Source: CAD feature listing. Evaluate the final solid. Frame: model axes, mm. Give positions to 0.01 mm unless a question says otherwise; leave off trailing zeros. Order: outer loops, then holes, each group sorted by start corner. A loop starts at its lowest first (then second) coordinate and runs counter-clockwise, first axis right, second up. Notation, with made-up numbers: M 20.25,52 L 39.25,52 A32 ccw 39.25,91 Z; hole C 42,49.5 d3. An arc over 180 degrees is marked long. Answer as a JSON object with one key per item and string values. Group by question number.
1. Section query D-D (z = 5.25). Output: boundary loops of the cut face in (x, y).
2. Section query B-B (x = 16). Output: boundary loops of the cut face in (y, z).
3. Material intervals for L1, parallel to Y at x = -16, z = 1.3; L2, parallel to X at y = 18, z = 0.65; L3, parallel to Y at x = -15.5, z = 0.75, sorted ascending. Write a range as [from, to].
4. Section query A-A (y = 18). Output: boundary loops of the cut face in (x, z).
5. Section query C-C (y = 12.5). Output: boundary loops of the cut face in (x, z), plus the area to 3 significant figures.
6. Pin query (flat end, axial travel): P1, Ø6.5, axis at x = -16, y = -10, coming from the -Z side; P2, Ø3, axis at x = -16, y = 18, coming from the +Z side; P3, Ø3, axis at x = 10, z = 6, coming from the -Y side; P4, Ø11.5, axis at x = -2.5, y = 0.5, coming from the +Z side. Return the tip coordinate at first contact, or that it passes through.
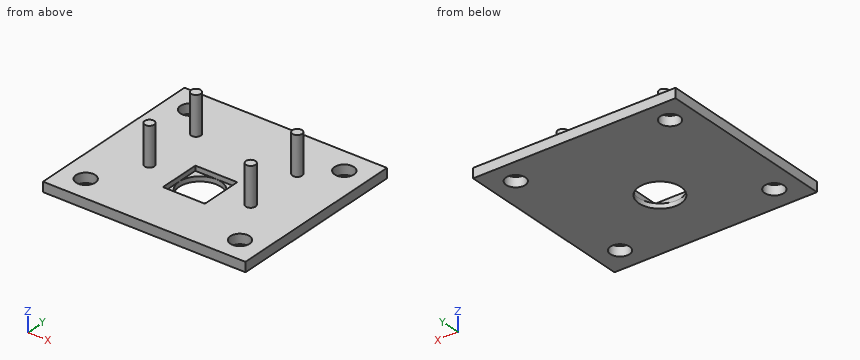
from build123d import *

# Parameters (mm, degrees)
CYLINDER002_R     = 1
CYLINDER002_DEPTH = 10
CYLINDER003_R     = 1
CYLINDER003_DEPTH = 10
CYLINDER004_R     = 1
CYLINDER004_DEPTH = 10
CYLINDER005_R     = 2
CYLINDER005_DEPTH = 10
CYLINDER006_R     = 2
CYLINDER006_DEPTH = 10
CYLINDER007_R     = 2
CYLINDER007_DEPTH = 10
CYLINDER008_R     = 2
CYLINDER008_DEPTH = 10
CYLINDER_R        = 4.35
CYLINDER_DEPTH    = 10
BOX_W             = 8.7
BOX_H             = 8.7
BOX_DEPTH         = 2
BOX001_W          = 42
BOX001_H          = 38
BOX001_DEPTH      = 2
CYLINDER001_R     = 1
CYLINDER001_DEPTH = 10


with BuildPart() as screw_support001:
    # Cylinder002 → Cylinder002 (new body)
    with BuildSketch(Plane(origin=(10.5, 0, 0), x_dir=(1, 0, 0), z_dir=(0, 0, 1))):
        Circle(CYLINDER002_R)
    extrude(amount=CYLINDER002_DEPTH)


with BuildPart() as screw_support002:
    # Cylinder003 → Cylinder003 (new body)
    with BuildSketch(Plane(origin=(-10.5, 12.5, 0), x_dir=(1, 0, 0), z_dir=(0, 0, 1))):
        Circle(CYLINDER003_R)
    extrude(amount=CYLINDER003_DEPTH)


with BuildPart() as screw_support003:
    # Cylinder004 → Cylinder004 (new body)
    with BuildSketch(Plane(origin=(10.5, 12.5, 0), x_dir=(1, 0, 0), z_dir=(0, 0, 1))):
        Circle(CYLINDER004_R)
    extrude(amount=CYLINDER004_DEPTH)


with BuildPart() as bolthole:
    # Cylinder005 → Cylinder005 (new body)
    with BuildSketch(Plane(origin=(-16, -10, 0), x_dir=(1, 0, 0), z_dir=(0, 0, 1))):
        Circle(CYLINDER005_R)
    extrude(amount=CYLINDER005_DEPTH)


with BuildPart() as bolthole001:
    # Cylinder006 → Cylinder006 (new body)
    with BuildSketch(Plane(origin=(16, 18, 0), x_dir=(1, 0, 0), z_dir=(0, 0, 1))):
        Circle(CYLINDER006_R)
    extrude(amount=CYLINDER006_DEPTH)


with BuildPart() as bolthole002:
    # Cylinder007 → Cylinder007 (new body)
    with BuildSketch(Plane(origin=(16, -10, 0), x_dir=(1, 0, 0), z_dir=(0, 0, 1))):
        Circle(CYLINDER007_R)
    extrude(amount=CYLINDER007_DEPTH)


with BuildPart() as bolthole003:
    # Cylinder008 → Cylinder008 (new body)
    with BuildSketch(Plane(origin=(-16, 18, 0), x_dir=(1, 0, 0), z_dir=(0, 0, 1))):
        Circle(CYLINDER008_R)
    extrude(amount=CYLINDER008_DEPTH)


with BuildPart() as cylinder:
    # Cylinder → Cylinder (new body)
    with BuildSketch(Plane.XY.offset(-3)):
        Circle(CYLINDER_R)
    extrude(amount=CYLINDER_DEPTH)


with BuildPart() as cube:
    # Box → Box (new body)
    with BuildSketch(Plane(origin=(-4.35, -4.35, 1), x_dir=(1, 0, 0), z_dir=(0, 0, 1))):
        with Locations((4.35, 4.35)):
            Rectangle(BOX_W, BOX_H)
    extrude(amount=BOX_DEPTH)


with BuildPart() as cut005:
    # Box001 → Box001 (new body)
    with BuildSketch(Plane(origin=(-21, -15, 0), x_dir=(1, 0, 0), z_dir=(0, 0, 1))):
        with Locations((21, 19)):
            Rectangle(BOX001_W, BOX001_H)
    extrude(amount=BOX001_DEPTH)

    # Cut: cut Cube
    add(cube.part, mode=Mode.SUBTRACT)

    # Cut001: cut Cylinder
    add(cylinder.part, mode=Mode.SUBTRACT)

    # Cut002: cut BoltHole003
    add(bolthole003.part, mode=Mode.SUBTRACT)

    # Cut003: cut BoltHole002
    add(bolthole002.part, mode=Mode.SUBTRACT)

    # Cut004: cut BoltHole001
    add(bolthole001.part, mode=Mode.SUBTRACT)

    # Cut005: cut BoltHole
    add(bolthole.part, mode=Mode.SUBTRACT)


with BuildPart() as fusion_camfront:
    # Cylinder001 → Cylinder001 (new body)
    with BuildSketch(Plane(origin=(-10.5, 0, 0), x_dir=(1, 0, 0), z_dir=(0, 0, 1))):
        Circle(CYLINDER001_R)
    extrude(amount=CYLINDER001_DEPTH)

    # Fusion: union screw support001, screw support002, screw support003, Cut005
    add(screw_support001.part)
    add(screw_support002.part)
    add(screw_support003.part)
    add(cut005.part)


solid = fusion_camfront.part
Answer sheet:
{
 "1": {"outline": "C -10.5,0 d2; C -10.5,12.5 d2; C 10.5,0 d2; C 10.5,12.5 d2"},
 "2": {"outline": "M -15,0 L -12,0 L -12,2 L -15,2 Z; M -8,0 L 16,0 L 16,2 L -8,2 Z; M 20,0 L 23,0 L 23,2 L 20,2 Z"},
 "3": {"L1": "[-15, -12], [-8, 16], [20, 23]", "L2": "[-21, -18], [-14, 14], [18, 21]", "L3": "[-15, -11.94], [-8.06, 16.06], [19.94, 23]"},
 "4": {"outline": "M -21,0 L -18,0 L -18,2 L -21,2 Z; M -14,0 L 14,0 L 14,2 L -14,2 Z; M 18,0 L 21,0 L 21,2 L 18,2 Z"},
 "5": {"outline": "M -21,0 L 21,0 L 21,2 L 11.5,2 L 11.5,10 L 9.5,10 L 9.5,2 L -9.5,2 L -9.5,10 L -11.5,10 L -11.5,2 L -21,2 Z", "area": "116 mm^2"},
 "6": {"P1": "z = 0", "P2": "through", "P3": "y = -1", "P4": "z = 2"}
}
